from build123d import *

# Parameters (mm, degrees)
PAD006_DEPTH = 0.3
FILLET005_R  = 0.1


with BuildPart() as part:
    # Sketch007 → Pad006 (new body, symmetric)
    with BuildSketch(Plane.XZ):
        Polygon((-4, 0), (-4, 0.1), (-3.7, 0.1), (-3.3, 0.5), (0, 0.5), (0, 0.4), (-3.258579, 0.4), (-3.658579, 0), align=None)
    pad006 = extrude(amount=PAD006_DEPTH, both=True)

    # Mirrored: Pad006 across Sketch007 V_Axis
    add(pad006.mirror(Plane(origin=(0, 0, 0), x_dir=(0, -1, 0), z_dir=(1, 0, 0))))

    # Fillet005
    fillet005_edges = [part.edges().sort_by_distance(p)[0] for p in [
        (-3.7, 0, 0.1),
        (-3.3, 0, 0.5),
        (-3.658579, 0, 0),
        (-3.258579, 0, 0.4),
        (3.258579, 0, 0.4),
        (3.658579, 0, 0),
        (3.3, 0, 0.5),
        (3.7, 0, 0.1),
    ]]
    fillet(fillet005_edges, radius=FILLET005_R)


solid = part.part
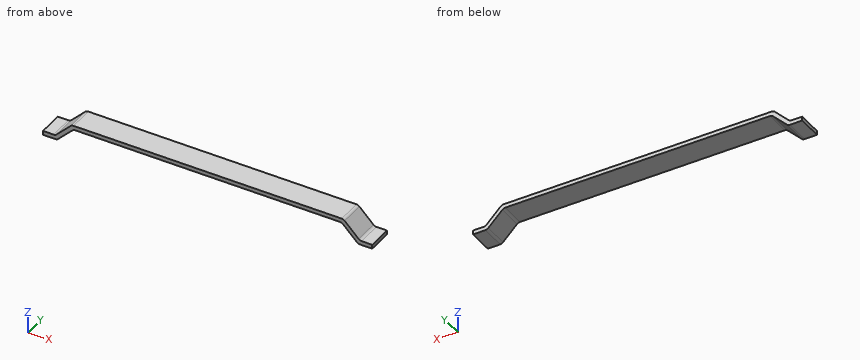
For this review, take the finished solid that the model builds, in its own axes (mm). Give positions to 0.01 mm unless a question says otherwise; leave off trailing zeros. Loops run counter-clockwise (first coordinate to the right, second up) from the corner with the lowest first, then second, coordinate; pieces in that order, holes last. Notation, with made-up numbers: M 76.5,42 L 90.5,42 A31 cw 90.5,75 Z; hole C 48.5,23 d7. An arc over 180 degrees is marked long. Answer as a JSON object with one key per item and string values. Group by question number.
Q1. Add section A-A on y = -0.1. Give the boundary of the cut face in (x, z), and give its area (3 significant figures).
Q2. Add section C-C on x = -0.5. Give the boundary of the cut face in (y, z), and give its area (3 significant figures).
Q3. Add section B-B on z = 0.25. Give the boundary of the cut face in (x, y).
Q4. For probe 1 along X at (y, z) = (-0.1, 0.45), list the stretches that pass through material, from the lowest coordinate up. Write a range as [from, to].
Q5. Add section D-D on x = -3.5. Give the boundary of the cut face in (y, z).
Checked values:
{
 "1": {"outline": "M -4,0 L -3.7,0 A0.1 ccw -3.63,0.03 L -3.29,0.37 A0.1 cw -3.22,0.4 L 3.22,0.4 A0.1 cw 3.29,0.37 L 3.63,0.03 A0.1 ccw 3.7,0 L 4,0 L 4,0.1 L 3.74,0.1 A0.1 cw 3.67,0.13 L 3.33,0.47 A0.1 ccw 3.26,0.5 L -3.26,0.5 A0.1 ccw -3.33,0.47 L -3.67,0.13 A0.1 cw -3.74,0.1 L -4,0.1 Z", "area": "0.833 mm²"},
 "2": {"outline": "M -0.3,0.4 L 0.3,0.4 L 0.3,0.5 L -0.3,0.5 Z", "area": "0.0600 mm²"},
 "3": {"outline": "M -3.55,-0.3 L -3.41,-0.3 L -3.41,0.3 L -3.55,0.3 Z; M 3.41,-0.3 L 3.55,-0.3 L 3.55,0.3 L 3.41,0.3 Z"},
 "4": {"probe 1": "[-3.35, 3.35]"},
 "5": {"outline": "M -0.3,0.16 L 0.3,0.16 L 0.3,0.3 L -0.3,0.3 Z"}
}
